from build123d import *

# Parameters (mm, degrees)
SKETCH1_W           = 203.2
SKETCH1_H           = 254
BOSS_EXTRUDE1_DEPTH = 3.175
SKETCH2_W           = 228.6
SKETCH2_H           = 47.625
BOSS_EXTRUDE2_DEPTH = 3.175
FILLET1_R           = 3.175


with BuildPart() as part:
    # Sketch1 → Boss-Extrude1 (new body)
    with BuildSketch(Plane(origin=(0, 0, 0), x_dir=(1, 0, 0), z_dir=(0, 1, 0))):
        with Locations((101.6, -127)):
            Rectangle(SKETCH1_W, SKETCH1_H)
    extrude(amount=BOSS_EXTRUDE1_DEPTH)

    # Sketch2 → Boss-Extrude2 (add, through all)
    with BuildSketch(Plane(origin=(0, 3.175, 0), x_dir=(1, 0, 0), z_dir=(0, 1, 0))):
        with Locations((101.6, -76.2)):
            Rectangle(SKETCH2_W, SKETCH2_H)
        with Locations((101.6, -177.8)):
            Rectangle(SKETCH2_W, SKETCH2_H)
    extrude(amount=-BOSS_EXTRUDE2_DEPTH)

    # Fillet1
    fillet1_edges = [part.edges().sort_by_distance(p)[0] for p in [
        (215.9, 1.5875, 100.0125),
        (-12.7, 1.5875, 52.3875),
        (215.9, 1.5875, 52.3875),
        (0, 1.5875, 100.0125),
        (203.2, 1.5875, 100.0125),
        (-12.7, 1.5875, 100.0125),
        (0, 1.5875, 52.3875),
        (203.2, 1.5875, 52.3875),
        (215.9, 1.5875, 201.6125),
        (-12.7, 1.5875, 153.9875),
        (215.9, 1.5875, 153.9875),
        (0, 1.5875, 201.6125),
        (203.2, 1.5875, 201.6125),
        (-12.7, 1.5875, 201.6125),
        (0, 1.5875, 153.9875),
        (203.2, 1.5875, 153.9875),
    ]]
    fillet(fillet1_edges, radius=FILLET1_R)


solid = part.part
For this review, take the finished solid that the model builds, in its own axes (mm). Round coordinates to 2 decimals unless told otherwise and drop trailing zeros. Loops run counter-clockwise (first coordinate to the right, second up) from the corner with the lowest first, then second, coordinate; pieces in that order, holes last. Notation, with made-up numbers: (-5, 75) - (40, 75) arc R20 cw to (40, 100) - close; hole circle Ø2 at (-26, 35). An arc over 180 degrees is marked (long way). One line per item, written item: value. Start each with the question number.
Item 1: Take a section at A-A (z = 20). Give the boundary of the cut face in (x, y) (3 decimals).
Item 2: Clearance check with flat-ended pins moving along their axes: pin 1 Ø1 at (y, z) = (1, 34) entering from +X; pin 2 Ø1 at (x, y) = (210.5, 1.5) entering from +Z; pin 3 Ø1 at (x, y) = (164.5, 2.5) entering from -Z; pin 4 Ø1.6 at (x, y) = (209.5, 1) entering from -Z. State where each tip first meets the part, or that it passes through.
Item 3: For L1, parallel to X at y = 3, z = 146; L2, parallel to X at y = 2.1, z = 153; L3, parallel to Z at x = 204, y = 3.05, list the stretches that pass through material, from the lowest coordinate up.
Answer below:
1. outline: (0, 0) - (203.2, 0) - (203.2, 3.175) - (0, 3.175) - close
2. pin 1: stops at x = 203.2
2. pin 2: stops at z = 201.61
2. pin 3: stops at z = 0
2. pin 4: stops at z = 52.39
3. L1: x = 0 to 203.2
3. L2: x = -0.87 to 204.07
3. L3: z = 51.32 to 101.08, 152.92 to 202.68
